Verification items for the finished model (mm, model axes). A direction names the side the tool comes from. Round coordinates to 2 decimals unless told otherwise and drop trailing zeros. Write each loop counter-clockwise with the first axis right and the second up, starting at its lowest first coordinate (ties: lowest second). Pieces come first, ordered by that corner, then holes. Notation, with made-up numbers: M 28,56 L 36,56 A33 ccw 36,95 Z; hole C 86.5,28.25 d9. An arc over 180 degrees is marked long. One line per question, with ' | ' between items. Start each with the question number.
Q1. Thickness scan on line 1 along Z through (x, y) = (0, 23); line 2 along X through (y, z) = (10, -1.5); line 3 along Z through (x, y) = (4, 13.5). Record the ranges inside material, lowest first. Write a range as from..to.
Q2. Gauge pin test, flat ends, axial feed: pin 1 (12 mm diameter, centred on x = -17.5, z = -27.5, fed in from +Y); pin 2 (4 mm diameter, centred on x = 0, z = 46.6, fed in from +Y); pin 3 (10 mm diameter, centred on x = -17, z = -27, fed in from +Y); pin 4 (10 mm diameter, centred on y = 6, z = 10, fed in from -X). Record the tip position at first contact, or that the pin passes through.
Q3. Release check for a two-part mould opening along Y. For faces 1 (the face through (27.12, 5.31, 17.93)), 2 (the face through (-10, 18, 40)), 3 (the face through (24.746, 14.79, 38.645)) record: released by +Y, released by -Y, zero draft, split by the parting line, or undercut.
Q4. Cross-section at B-B (z = -10.5). Record the boundary of the cut face in (x, y).
Q5. Cross-section at C-C (z = 27.5). Record the boundary of the cut face in (x, y).
Q6. Tool access check on faces 4 (the face through (0, 16, -38.1)), 5 (the face through (31.7, 2.03, 15.14)), 6 (the face through (0.2, 25, 44.7)). Record the directions out of +Z, -Z, +X, -X, +Y, -Y that give a thin tool (end or side, any length) a straight path to the whole face; none if there is none.
Q7. Cross-section at A-A (y = 15). State how many separate pieces and enclosed holes the cut face has, then the cut area to 3 significant figures.
from build123d import *

# Parameters (mm, degrees)
BOSS_EXTRUDE1_DEPTH      = 30
BOSS_EXTRUDE2_DEPTH      = 27
BOSS_EXTRUDE3_DEPTH      = 2.5
FILLET1_R                = 3
BORNIER_REACH            = 92.559
SKETCH3_R                = 2
BOSS_EXTRUDE4_DEPTH      = 4
FILLET2_R                = 3
FILLET3_R                = 7
BOSS_EXTRUDE6_DEPTH      = 10
BOSS_EXTRUDE6_DEPTH_BACK = 10
SKETCH5_R                = 1.65
SKETCH5_R_2              = 1
CUT_EXTRUDE2_DEPTH       = 70.28195973
CUT_EXTRUDE2_DEPTH_BACK  = 70.28195973
SKETCH6_W                = 10.000691042
SKETCH6_H                = 10
FILLET4_R                = 3
CUT_EXTRUDE3_DEPTH       = 1.5
CUT_EXTRUDE4_REACH       = 95.984
SKETCH7_3_W              = 4
SKETCH7_3_H              = 6
FILLET5_R                = 2


# Some blends are built 0.0001 mm under size
with BuildPart() as part:
    # Sketch1 → Boss-Extrude1 (new body)
    with BuildSketch(Plane(origin=(0, 0, 0), x_dir=(1, 0, 0), z_dir=(0, 1, 0))):
        with BuildLine():
            Line((-20.1, 40.6), (20.1, 40.6))
            ThreePointArc((20.1, 40.6), (24.696194078, 38.696194078), (26.6, 34.1))
            Line((26.6, 34.1), (26.6, -34.1))
            ThreePointArc((26.6, -34.1), (24.696194078, -38.696194078), (20.1, -40.6))
            Line((20.1, -40.6), (-20.1, -40.6))
            ThreePointArc((-20.1, -40.6), (-24.696194078, -38.696194078), (-26.6, -34.1))
            Line((-26.6, -34.1), (-26.6, 34.1))
            ThreePointArc((-26.6, 34.1), (-24.696194078, 38.696194078), (-20.1, 40.6))
        make_face()
        with BuildLine():
            ThreePointArc((-20.1, 39.1), (-23.635533906, 37.635533906), (-25.1, 34.1))
            Line((-25.1, 34.1), (-25.1, -34.1))
            ThreePointArc((-25.1, -34.1), (-23.635533906, -37.635533906), (-20.1, -39.1))
            Line((-20.1, -39.1), (20.1, -39.1))
            ThreePointArc((20.1, -39.1), (23.635533906, -37.635533906), (25.1, -34.1))
            Line((25.1, -34.1), (25.1, 34.1))
            ThreePointArc((25.1, 34.1), (23.635533906, 37.635533906), (20.1, 39.1))
            Line((20.1, 39.1), (-20.1, 39.1))
        make_face(mode=Mode.SUBTRACT)
    extrude(amount=BOSS_EXTRUDE1_DEPTH)

    # Sketch1<3> → Boss-Extrude2 (add)
    with BuildSketch(Plane(origin=(0, 0, 0), x_dir=(1, 0, 0), z_dir=(0, 1, 0))):
        with BuildLine():
            Line((-20.1, 39.1), (20.1, 39.1))
            ThreePointArc((20.1, 39.1), (23.635533906, 37.635533906), (25.1, 34.1))
            Line((25.1, 34.1), (25.1, -34.1))
            ThreePointArc((25.1, -34.1), (23.635533906, -37.635533906), (20.1, -39.1))
            Line((20.1, -39.1), (-20.1, -39.1))
            ThreePointArc((-20.1, -39.1), (-23.635533906, -37.635533906), (-25.1, -34.1))
            Line((-25.1, -34.1), (-25.1, 34.1))
            ThreePointArc((-25.1, 34.1), (-23.635533906, 37.635533906), (-20.1, 39.1))
        make_face()
        with BuildLine():
            ThreePointArc((-20.1, 38.1), (-22.928427125, 36.928427125), (-24.1, 34.1))
            Line((-24.1, 34.1), (-24.1, -34.1))
            ThreePointArc((-24.1, -34.1), (-22.928427125, -36.928427125), (-20.1, -38.1))
            Line((-20.1, -38.1), (20.1, -38.1))
            ThreePointArc((20.1, -38.1), (22.928427125, -36.928427125), (24.1, -34.1))
            Line((24.1, -34.1), (24.1, 34.1))
            ThreePointArc((24.1, 34.1), (22.928427125, 36.928427125), (20.1, 38.1))
            Line((20.1, 38.1), (-20.1, 38.1))
        make_face(mode=Mode.SUBTRACT)
    extrude(amount=BOSS_EXTRUDE2_DEPTH)

    # Sketch1<4> → Boss-Extrude3 (add)
    with BuildSketch(Plane(origin=(0, 0, 0), x_dir=(1, 0, 0), z_dir=(0, 1, 0))):
        with BuildLine():
            Line((-20.1, 38.1), (20.1, 38.1))
            ThreePointArc((20.1, 38.1), (22.928427125, 36.928427125), (24.1, 34.1))
            Line((24.1, 34.1), (24.1, -34.1))
            ThreePointArc((24.1, -34.1), (22.928427125, -36.928427125), (20.1, -38.1))
            Line((20.1, -38.1), (-20.1, -38.1))
            ThreePointArc((-20.1, -38.1), (-22.928427125, -36.928427125), (-24.1, -34.1))
            Line((-24.1, -34.1), (-24.1, 34.1))
            ThreePointArc((-24.1, 34.1), (-22.928427125, 36.928427125), (-20.1, 38.1))
        make_face()
    extrude(amount=BOSS_EXTRUDE3_DEPTH)

    # Fillet1
    fillet1_edges = [part.edges().sort_by_distance(p)[0] for p in [
        (22.928427125, 2.5, 36.928427125),
        (-22.928427125, 2.5, -36.928427125),
        (0, 2.5, 38.1),
        (24.1, 2.5, 0),
        (22.928427125, 2.5, -36.928427125),
        (0, 2.5, -38.1),
        (-24.1, 2.5, 0),
        (-22.928427125, 2.5, 36.928427125),
    ]]
    fillet(fillet1_edges, radius=FILLET1_R)

    # Sketch3 → Bornier (cut, up to next)
    with BuildSketch(Plane(origin=(0, 0, -40.6), x_dir=(-1, 0, 0), z_dir=(0, 0, -1)), mode=Mode.PRIVATE) as bornier_sk1:
        with Locations((-10, 15)):
            Circle(SKETCH3_R)
    bornier_tool1 = extrude(bornier_sk1.sketch, amount=-BORNIER_REACH, mode=Mode.PRIVATE) & part.part
    # Sketch3 → Bornier (cut, up to next)
    with BuildSketch(Plane(origin=(0, 0, -40.6), x_dir=(-1, 0, 0), z_dir=(0, 0, -1)), mode=Mode.PRIVATE) as bornier_sk2:
        with Locations((10, 15)):
            Circle(SKETCH3_R)
    bornier_tool2 = extrude(bornier_sk2.sketch, amount=-BORNIER_REACH, mode=Mode.PRIVATE) & part.part
    add(bornier_tool1.solids().sort_by_distance((10, 15, -40.6))[0], mode=Mode.SUBTRACT)
    add(bornier_tool2.solids().sort_by_distance((-10, 15, -40.6))[0], mode=Mode.SUBTRACT)

    # Sketch4 → Boss-Extrude4 (add)
    with BuildSketch(Plane.XZ):
        Polygon((26.6, 16), (32.6, 16), (32.6, -16), (26.6, -16), (26.6, -20), (36.6, -20), (36.6, 20), (26.6, 20), align=None)
        Polygon((-26.6, 16), (-26.6, 20), (-36.6, 20), (-36.6, -20), (-26.6, -20), (-26.6, -16), (-32.6, -16), (-32.6, 16), align=None)
    extrude(amount=-BOSS_EXTRUDE4_DEPTH)

    # Fillet2
    fillet2_edges = [part.edges().sort_by_distance(p)[0] for p in [
        (32.6, 2, 16),
        (32.6, 2, -16),
        (26.6, 2, -20),
        (26.6, 2, -16),
        (26.6, 4, -18),
        (26.6, 4, 18),
        (26.6, 2, 20),
        (26.6, 2, 16),
        (-32.6, 2, -16),
        (-26.6, 2, -20),
        (-26.6, 4, -18),
        (-26.6, 2, -16),
        (-26.6, 4, 18),
        (-26.6, 2, 20),
        (-26.6, 2, 16),
        (-32.6, 2, 16),
    ]]
    fillet(fillet2_edges, radius=FILLET2_R - 0.0001)  # a hair under: the kernel refuses the full size

    # Fillet3
    fillet3_edges = [part.edges().sort_by_distance(p)[0] for p in [
        (-36.6, 2, -20),
        (-36.6, 2, 20),
        (36.6, 2, -20),
        (36.6, 2, 20),
    ]]
    fillet(fillet3_edges, radius=FILLET3_R)

    # Sketch5 → Boss-Extrude6 (add, two sides: drawn at the far end of the back side and taken through both)
    with BuildSketch(Plane(origin=(0, 15, 0), x_dir=(-1, 0, 0), z_dir=(0, -1, 0)).offset(-BOSS_EXTRUDE6_DEPTH_BACK)):
        with BuildLine():
            Line((16.522711642, -40.6), (-16.522711642, -40.6))
            ThreePointArc((-16.522711642, -40.6), (-15.897493185, -42.62243393), (-15.025773528, -44.551486018))
            add(Edge.make_bspline(
                [(-15.025773528, -44.551486018), (-14.228677761, -46.057742891), (-9.345567408, -49.968366267), (-3.844651769, -50.600691042), (0, -50.600691042)],
                knots=[0, 0, 0, 0, 0.327378903, 1, 1, 1, 1], degree=3))
            add(Edge.make_bspline(
                [(15.025773528, -44.551486018), (14.228677761, -46.057742891), (9.345567408, -49.968366267), (3.844651769, -50.600691042), (0, -50.600691042)],
                knots=[0, 0, 0, 0, 0.327378903, 1, 1, 1, 1], degree=3))
            ThreePointArc((15.025773528, -44.551486018), (15.897493185, -42.62243393), (16.522711642, -40.6))
        make_face()
        with Locations(Location((0, -46.6, 0), (0, 0, 90))):
            Circle(SKETCH5_R, mode=Mode.SUBTRACT)
        with Locations(Location((-5.977168189, -46.077065544, 0), (0, 0, 90))):
            Circle(SKETCH5_R_2, mode=Mode.SUBTRACT)
        with Locations(Location((-10.958141679, -45.64128683, 0), (0, 0, 90))):
            Circle(SKETCH5_R_2, mode=Mode.SUBTRACT)
        with Locations(Location((10.958141679, -45.64128683, 0), (0, 0, 270))):
            Circle(SKETCH5_R_2, mode=Mode.SUBTRACT)
        with Locations(Location((5.977168189, -46.077065544, 0), (0, 0, 270))):
            Circle(SKETCH5_R_2, mode=Mode.SUBTRACT)
    extrude(amount=BOSS_EXTRUDE6_DEPTH + BOSS_EXTRUDE6_DEPTH_BACK)

    # Sketch6 → Cut-Extrude2 (cut, two sides: drawn at the far end of the back side and taken through both)
    with BuildSketch(Plane(origin=(0, 0, 0), x_dir=(0, 0, -1), z_dir=(1, 0, 0)).offset(-CUT_EXTRUDE2_DEPTH_BACK)):
        with Locations((-45.600345521, 15)):
            Rectangle(SKETCH6_W, SKETCH6_H)
    extrude(amount=CUT_EXTRUDE2_DEPTH + CUT_EXTRUDE2_DEPTH_BACK, mode=Mode.SUBTRACT)

    # Fillet4
    fillet4_edges = [part.edges().sort_by_distance(p)[0] for p in [
        (-16.522711642, 22.5, 40.6),
        (16.522711642, 22.5, 40.6),
        (0, 25, 40.6),
        (0, 5, 40.6),
        (16.522711642, 7.5, 40.6),
        (-16.522711642, 7.5, 40.6),
    ]]
    fillet(fillet4_edges, radius=FILLET4_R)

    # Sketch7 → Cut-Extrude3 (cut)
    with BuildSketch(Plane.XY.offset(40.6)):
        with BuildLine():
            Line((-6.020797289, 18), (-13, 18))
            Line((-13, 18), (-13, 12))
            Line((-13, 12), (-6.020797289, 12))
            ThreePointArc((-6.020797289, 12), (-4.870349806, 11.770644436), (-3.895810011, 11.117647059))
            ThreePointArc((-3.895810011, 11.117647059), (5.5, 15), (-3.895810011, 18.882352941))
            ThreePointArc((-3.895810011, 18.882352941), (-4.870349806, 18.229355564), (-6.020797289, 18))
        make_face()
    extrude(amount=-CUT_EXTRUDE3_DEPTH, mode=Mode.SUBTRACT)

    # Sketch7<3> → Cut-Extrude4 (cut, up to next)
    with BuildSketch(Plane.XY.offset(40.6), mode=Mode.PRIVATE) as cut_extrude4_sk1:
        with Locations((-11, 15)):
            Rectangle(SKETCH7_3_W, SKETCH7_3_H)
    cut_extrude4_tool1 = extrude(cut_extrude4_sk1.sketch, amount=-CUT_EXTRUDE4_REACH, mode=Mode.PRIVATE) & part.part
    add(cut_extrude4_tool1.solids().sort_by_distance((-11, 15, 40.6))[0], mode=Mode.SUBTRACT)

    # Fillet5
    # the kernel refuses this fillet: 2 mm, written as the material it takes off along each edge
    with BuildSketch(Plane(origin=(-7.291287847, 10, 40.6), x_dir=(0, 0, 1), z_dir=(1, 0, 0))) as fillet5_piece_1_section:
        with BuildLine():
            CenterArc((FILLET5_R, FILLET5_R), FILLET5_R, 180, 90)
            Line((0, FILLET5_R), (-FILLET5_R * 0.02, FILLET5_R))
            Line((-FILLET5_R * 0.02, FILLET5_R), (-FILLET5_R * 0.02, -FILLET5_R * 0.02))
            Line((-FILLET5_R * 0.02, -FILLET5_R * 0.02), (FILLET5_R, -FILLET5_R * 0.02))
            Line((FILLET5_R, -FILLET5_R * 0.02), (FILLET5_R, 0))
        make_face()
    fillet5_piece_1 = extrude(amount=14.582575695, mode=Mode.PRIVATE)
    fillet5_piece_1 = split(fillet5_piece_1, bisect_by=Plane(origin=(-1.49e-07, 9.863484185, 40.6), z_dir=(0, 0, 1)), keep=Keep.TOP, mode=Mode.PRIVATE)
    fillet5_piece_1 = fillet5_piece_1 & Plane(origin=(0, 15, 41.29634072), x_dir=(-0.708329092870135, -0.7058823529411764, 0), z_dir=(0, 0, 1)) * Cylinder(5.5, 38, mode=Mode.PRIVATE)
    add(fillet5_piece_1, mode=Mode.SUBTRACT)
    with BuildSketch(Plane(origin=(7.291287847, 20, 40.6), x_dir=(0, 1, 0), z_dir=(-1, 0, 0))) as fillet5_piece_2_section:
        with BuildLine():
            CenterArc((FILLET5_R, -FILLET5_R), FILLET5_R, 90, 90)
            Line((0, -FILLET5_R), (-FILLET5_R * 0.02, -FILLET5_R))
            Line((-FILLET5_R * 0.02, -FILLET5_R), (-FILLET5_R * 0.02, FILLET5_R * 0.02))
            Line((-FILLET5_R * 0.02, FILLET5_R * 0.02), (FILLET5_R, FILLET5_R * 0.02))
            Line((FILLET5_R, FILLET5_R * 0.02), (FILLET5_R, 0))
        make_face()
    fillet5_piece_2 = extrude(amount=14.582575695, mode=Mode.PRIVATE)
    fillet5_piece_2 = split(fillet5_piece_2, bisect_by=Plane(origin=(1.13e-07, 20.136515828, 40.6), z_dir=(0, 0, 1)), keep=Keep.TOP, mode=Mode.PRIVATE)
    fillet5_piece_2 = fillet5_piece_2 & Plane(origin=(0, 15, 41.29634056), x_dir=(-0.708329092870135, -0.7058823529411764, 0), z_dir=(0, 0, 1)) * Cylinder(5.5, 38, mode=Mode.PRIVATE)
    add(fillet5_piece_2, mode=Mode.SUBTRACT)


solid = part.part
Determined:
1) line 1: z = -40.6..-38.1, 38.1..44.95, 48.25..50.6 | line 2: x = -26.6..-24.1, 24.1..26.6 | line 3: z = -40.6..-38.1, 38.1..39.1
2) pin 1: stops at y = 3.7 | pin 2: stops at y = 25 | pin 3: stops at y = 2.64 | pin 4: stops at x = -36.6
3) face 1: released by +Y | face 2: undercut | face 3: zero draft
4) outline: M -36.6,0 L -32.6,0 L -32.6,4 L -36.6,4 Z; M -26.6,0 L 26.6,0 L 26.6,30 L 25.1,30 L 25.1,27 L 24.1,27 L 24.1,5.5 A3 cw 21.1,2.5 L -21.1,2.5 A3 cw -24.1,5.5 L -24.1,27 L -25.1,27 L -25.1,30 L -26.6,30 Z; M 32.6,0 L 36.6,0 L 36.6,4 L 32.6,4 Z
5) outline: M -26.6,0 L 26.6,0 L 26.6,30 L 25.1,30 L 25.1,27 L 24.1,27 L 24.1,5.5 A3 cw 21.1,2.5 L -21.1,2.5 A3 cw -24.1,5.5 L -24.1,27 L -25.1,27 L -25.1,30 L -26.6,30 Z
6) face 4: +Y | face 5: +Y, -Y | face 6: +Z, +X, -X, +Y
7) separate pieces: 3 | enclosed holes: 0 | area: 573 mm²
